Read the model definition and answer for the solid it produces. Units are mm, in the model's axes. Give positions to 0.01 mm unless a question says otherwise; leave off trailing zeros. Order: outer loops, then holes, each group sorted by start corner. A loop starts at its lowest first (then second) coordinate and runs counter-clockwise, first axis right, second up. Notation, with made-up numbers: (15, 10.25) - (55, 10.25) arc R19 ccw to (55, 26.25) - close; hole circle Ø8 at (-9.5, 31.5). An arc over 180 degrees is marked (long way). Return JSON: item names as keys, results as strings.
```python
from build123d import *

# Parameters (mm, degrees)
SKETCH1_W           = 40
SKETCH1_H           = 4
BOSS_EXTRUDE1_DEPTH = 34
SKETCH2_R           = 1.5
CUT_EXTRUDE1_DEPTH  = 6
SKETCH3_W           = 4
SKETCH3_H           = 34
BOSS_EXTRUDE2_DEPTH = 22
BOSS_EXTRUDE3_DEPTH = 4


with BuildPart() as part:
    # Sketch1 → Boss-Extrude1 (new body)
    with BuildSketch(Plane(origin=(0, 0, 0), x_dir=(1, 0, 0), z_dir=(0, 1, 0))):
        Rectangle(SKETCH1_W, SKETCH1_H)
    extrude(amount=BOSS_EXTRUDE1_DEPTH)

    # Sketch2 → Cut-Extrude1 (cut)
    with BuildSketch(Plane.XZ):
        Circle(SKETCH2_R)
    cut_extrude1 = extrude(amount=-CUT_EXTRUDE1_DEPTH, mode=Mode.SUBTRACT)

    # Mirror1: Cut-Extrude1 across plane
    add(cut_extrude1.mirror(Plane(origin=(0, 17, 0), x_dir=(0, 0, 1), z_dir=(0, -1, 0))), mode=Mode.SUBTRACT)

    # Sketch3 → Boss-Extrude2 (add)
    with BuildSketch(Plane.ZY.offset(20)):
        with Locations((0, 17)):
            Rectangle(SKETCH3_W, SKETCH3_H)
    extrude(amount=BOSS_EXTRUDE2_DEPTH)

    # Sketch5 → Boss-Extrude3 (add)
    with BuildSketch(Plane(origin=(0, 0, -2), x_dir=(-1, 0, 0), z_dir=(0, 0, -1))):
        Polygon((-20, 29.024641929), (42, 33), (42, 34), (-20, 34), align=None)
        Polygon((42, 0), (-20, 0), (-20, 4.975358071), (42, 1), align=None)
    extrude(amount=BOSS_EXTRUDE3_DEPTH)


solid = part.part
```
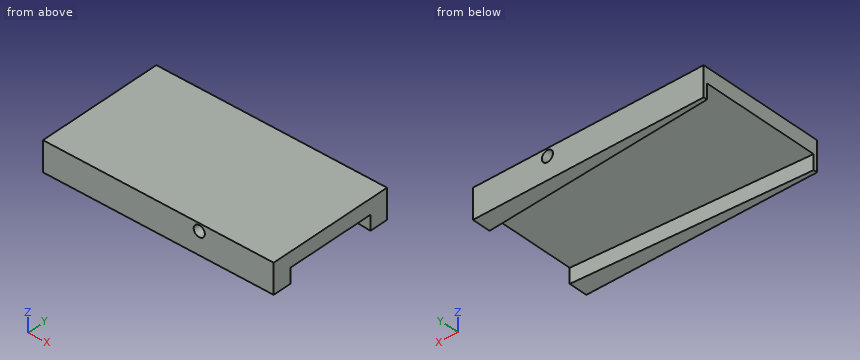
Q1. A cutting plane is placed at D-D (y = 17). Write down the section's boundary in (x, z), and give its area (3 significant figures).
Values:
{"outline": "(-42, -2) - (20, -2) - (20, 2) - (-42, 2) - close", "area": "248 mm²"}
Q2. A cutting plane is placed at A-A (z = -4.5). Write down the section's boundary in (x, y), and give its area (3 significant figures).
Values:
{"outline": "(-42, 0) - (20, 0) - (20, 4.98) - (-42, 1) - close; (-42, 33) - (20, 29.02) - (20, 34) - (-42, 34) - close", "area": "370 mm²"}
Q3. Given pin 1 (3 mm diameter, centred on x = -34, y = 19, fed in from -Z); pin 2 (1.8 mm diameter, centred on x = 0, z = 0, fed in from -Y), each flat-ended and moving along its own axis, determine where each tip first touches the part or whether it passes through.
Values:
{"pin 1": "stops at z = -2", "pin 2": "stops at y = 6"}
Q4. A cutting plane is placed at C-C (z = 0). Write down the section's boundary in (x, y).
Values:
{"outline": "(-42, 0) - (-1.5, 0) - (-1.5, 6) - (1.5, 6) - (1.5, 0) - (20, 0) - (20, 34) - (1.5, 34) - (1.5, 28) - (-1.5, 28) - (-1.5, 34) - (-42, 34) - close"}
Q5. Consider L1, parallel to Z at x = 0, y = 2.2; L2, parallel to Z at x = 0, y = 29; L3, parallel to Z at x = 17, y = 15. Determine where each line is inside the solid, lowest interval first.
Values:
{"L1": "z = -6 to -1.5, 1.5 to 2", "L2": "z = -2 to -1.5, 1.5 to 2", "L3": "z = -2 to 2"}
Q6. A cutting plane is placed at B-B (x = -0.5). Write down the section's boundary in (y, z).
Values:
{"outline": "(0, -6) - (3.66, -6) - (3.66, -2) - (30.34, -2) - (30.34, -6) - (34, -6) - (34, -1.41) - (28, -1.41) - (28, 1.41) - (34, 1.41) - (34, 2) - (0, 2) - (0, 1.41) - (6, 1.41) - (6, -1.41) - (0, -1.41) - close"}
